Source: CAD feature listing. Evaluate the final solid. Frame: model axes, mm. A direction names the side the tool comes from. Round coordinates to 2 decimals unless told otherwise and drop trailing zeros. Loops run counter-clockwise (first coordinate to the right, second up) from the corner with the lowest first, then second, coordinate; pieces in that order, holes last. Notation, with made-up numbers: (65, 15.25) -> (101, 15.25) arc R11 cw to (101, 23.25) -> close; hole circle Ø11 at (62.5, -40). An arc over 180 degrees is marked (long way). Put each result on its own line as item: value. Start each with the question number.
1. Material intervals for L1, parallel to Z at x = 0.85, y = 15; L2, parallel to Z at x = 1.35, y = 34; L3, parallel to Y at x = 0.2, z = 98, sorted ascending.
2. Cut plane B-B (z = 66.5). Return the cut outline in (x, y), then the cut area to 3 significant figures.
3. Set-up query: faces 1 (the flat face through (1, 75, 62)), 2 (the flat face through (1, 26.69, 85)). Return all of +Z, -Z, +X, -X, +Y, -Y with unobstructed straight access to the full face (end or side cutting, diameter ignored); none if empty.
4. Draft query along Z for faces 3 (the flat face through (1, 38, 125)), 4 (the flat face through (1, 28.444, 23)), 5 (the flat face through (1, 17, 8.89)), 6 (the flat face through (0, 45, 63)). Return one class per face: pulls with the +Z half, pulls with the -Z half, needs draft (parallel to the pull), parting line crosses it, or undercut.
5. Cut plane C-C (x = 0.45). Return the cut outline in (y, z).
6. Contact query for a flat-ended pin moving along its axis: pin 1 (12 mm diameter, centred on y = 31.5, z = 65.5, fed in from -X). Output: stop coordinate, or through.
7. Cut plane A-A (y = 34.5). Return the cut outline in (x, z).
8. Cut plane D-D (y = 47). Return the cut outline in (x, z).
```python
from build123d import *

# Parameters (mm, degrees)
F0_W     = 16.253128
F0_H     = 4.658509
F1_DEPTH = 2.5


with BuildPart() as f1:
    # F0 (on Right) → F1 (new body)
    with BuildSketch(Plane.YZ):
        Polygon((0, 125), (0, 0), (75, 0), (75, 125), (71.19, 125), (50.19, 125), (49.408, 125), (44.505585, 125), align=None)
        Polygon((50.19, 121.19), (71.19, 121.19), (71.19, 3.81), (3.81, 3.81), (3.81, 121.19), (44.505585, 121.19), (49.408, 121.19), align=None, mode=Mode.SUBTRACT)
        Polygon((71.19, 3.81), (71.19, 121.19), (50.19, 121.19), (49.408, 121.19), (44.505585, 121.19), (3.81, 121.19), (3.81, 3.81), align=None)
        Polygon((5.690006, 116.11), (48.26, 116.11), (48.26, 95.11), (26.690006, 95.11), (26.690006, 74.11), (42.943134, 74.11), (42.943134, 36.768509), (28.444385, 36.768509), (28.444385, 8.89), (5.690006, 8.89), (5.690006, 53.11), (5.690006, 57.768509), align=None, mode=Mode.SUBTRACT)
        with Locations((13.81657, 55.439254)):
            Rectangle(F0_W, F0_H)
    extrude(amount=F1_DEPTH)


solid = f1.part
```
Solution:
1. L1: z = 0 to 8.89, 53.11 to 57.77, 116.11 to 125
1. L2: z = 0 to 36.77, 74.11 to 95.11, 116.11 to 125
1. L3: y = 0 to 5.69, 48.26 to 75
2. outline: (0, 0) -> (2.5, 0) -> (2.5, 5.69) -> (0, 5.69) -> close; (0, 42.94) -> (2.5, 42.94) -> (2.5, 75) -> (0, 75) -> close
2. area: 94.4 mm^2
3. face 1: +Z, -Z, +X, -X, +Y
3. face 2: +X, -X
4. face 3: pulls with the +Z half
4. face 4: undercut
4. face 5: undercut
4. face 6: needs draft
5. outline: (0, 0) -> (75, 0) -> (75, 125) -> (0, 125) -> close; hole (5.69, 8.89) -> (28.44, 8.89) -> (28.44, 36.77) -> (42.94, 36.77) -> (42.94, 74.11) -> (26.69, 74.11) -> (26.69, 95.11) -> (48.26, 95.11) -> (48.26, 116.11) -> (5.69, 116.11) -> (5.69, 57.77) -> (21.94, 57.77) -> (21.94, 53.11) -> (5.69, 53.11) -> close
6. pin 1: passes through
7. outline: (0, 0) -> (2.5, 0) -> (2.5, 36.77) -> (0, 36.77) -> close; (0, 74.11) -> (2.5, 74.11) -> (2.5, 95.11) -> (0, 95.11) -> close; (0, 116.11) -> (2.5, 116.11) -> (2.5, 125) -> (0, 125) -> close
8. outline: (0, 0) -> (2.5, 0) -> (2.5, 95.11) -> (0, 95.11) -> close; (0, 116.11) -> (2.5, 116.11) -> (2.5, 125) -> (0, 125) -> close
